Part model, mm, in its own coordinate system. A direction names the side the tool comes from. Round coordinates to 2 decimals unless told otherwise and drop trailing zeros. Loops run counter-clockwise (first coordinate to the right, second up) from the corner with the lowest first, then second, coordinate; pieces in that order, holes last. Notation, with made-up numbers: M -38,82 L 16,82 A29 cw 16,103 Z; hole C 41.5,27.5 d11. An arc over 180 degrees is marked long. Put each result on its own line as item: value. Start each with the question number.
1) Which spindle directions (+Z, -Z, +X, -X, +Y, -Y) get a long thin tool onto all of the face, cutting with end or side? Do faces 1 (the cylindrical face through (15.893, 0.211, 14.444)), 2 (the cylindrical face through (0, 26, 6)), 3 (the cylindrical face through (-15.893, 0.211, -14.444)). Say none if no direction does.
2) Pull direction Y, two halves, no side cores. Call faces 4 (the cylindrical face through (3, 0, -26)), 5 (the flat face through (0, 0, -33.5)), 6 (the cylindrical face through (15.918, 0.351, -14.444)): +Y half, -Y half, draft (parallel to the pull), parting line (faces both ways), or undercut.
3) Probe line 1 along Z through (x, y) = (9, 6.5); line 2 along Y through (x, z) = (-16.5, 18); line 3 along Y through (x, z) = (17.5, 14). List the from-to ranges inside material, lowest first.
4) Slice it at C-C on y = 23. Give the cut face in (x, z), then the cut area to 3 significant figures.
5) Slice it at B-B on z = -16. Give the cut face in (x, y), then the cut area to 3 significant figures.
6) Drop flat-ended pins along their axis: pin 1 Ø12 at (x, y) = (4.5, 20) entering from -Z; pin 2 Ø1 at (x, y) = (7.5, 14.5) entering from +Z; pin 3 Ø10 at (x, z) = (10.5, -3) entering from +Y; pin 4 Ø10 at (y, z) = (20.5, -27) entering from +X. Give the stop position or say it passes through.
7) Slice it at A-A on x = 0. Give the cut face in (y, z).
8) Slice it at D-D on z = -22. Give the cut face in (x, y).
Autodesk Inventor part; units mm, degrees
ref_plane "Arbeitsebene1" through (0, 25, 0) normal (0, 1, 0) x (-1, 0, 0)
ref_plane "YZ Plane" through (0, 0, 0) normal (1, 0, 0) x (0, 1, 0)
ref_plane "XY Plane" through (0, 0, 0) normal (0, 0, 1) x (1, 0, 0)
sketch "Skizze1" plane through (0, 0, 0) normal (0, 0, 1) x (1, 0, 0)
  circle A0 centre (0, 0) radius 25
  dimension "d0" = 50
extrude "Extrusion1" add sketch "Skizze1" along normal mid plane 37
sketch "Skizze2" plane through (0, 0, 18.5) normal (0, 0, 1) x (1, 0, 0)
  circle A0 centre (0, 0) radius 25
  circle A1 centre (0, 0) radius 3
  dimension "d3" = 6
extrude "Extrusion2" add sketch "Skizze2" along normal blind 6 contours A1
sketch "Skizze3" plane through (0, 0, -18.5) normal (0, 0, -1) x (-1, 0, 0)
  circle A0 centre (0, 0) radius 25
  circle A1 centre (0, 0) radius 3
  dimension "d6" = 6
extrude "Extrusion3" add sketch "Skizze3" along normal blind 15 contours A1
chamfer "Fase1" distance 0.5 angle 45 2 edges at (3, 0, -33.5) (-3, 0, 24.5)
sketch "Skizze4" plane through (0, 0, 18.5) normal (0, 0, 1) x (1, 0, 0)
  circle A0 centre (0, 0) radius 3
  line L0 (-17.5, 0) -> (17.5, 0) construction
  dimension "d12" = 35
hole "Bohrung1" at (-17.5, 0, 18.5) at (17.5, 0, 18.5) direction (0, 0, -1) diameter 3.242 depth 8 tip angle 118
mirror "Spiegeln1" about plane through (0, 0, 0) normal (0, 0, 1) of "Bohrung1"
ref_plane "Arbeitsebene1" through (0, 25, 0) normal (0, 1, 0) x (-1, 0, 0)
sketch "Skizze5" plane through (0, 25, 0) normal (0, 1, 0) x (-1, 0, 0)
  line L0 (-25, -18.5) -> (25, -18.5)
  line L1 (25, 18.5) -> (-25, 18.5)
  circle A0 centre (0, 3.5) radius 2.5
  point P0 (0, 0)
  dimension "d20" = 15
  dimension "d21" = 5
extrude "Extrusion4" add sketch "Skizze5" against normal blind 2 and the other way blind 2
properties part number "Tunel_Motor"
Recorded:
1. face 1: +Z
1. face 2: +Y
1. face 3: -Z
2. face 4: parting line
2. face 5: draft
2. face 6: undercut
3. line 1: z = -18.5 to 18.5
3. line 2: y = -18.78 to -1.28, 1.28 to 18.78
3. line 3: y = -17.85 to -1.62, 1.62 to 17.85
4. outline: M -9.8,-18.5 L 9.8,-18.5 L 9.8,18.5 L -9.8,18.5 Z
4. area: 725 mm2
5. outline: C 0,0 d50; hole C -17.5,0 d3.24; hole C 17.5,0 d3.24
5. area: 1,950 mm2
6. pin 1: stops at z = -18.5
6. pin 2: stops at z = 18.5
6. pin 3: stops at y = 24.39
6. pin 4: passes through
7. outline: M -25,-18.5 L -3,-18.5 L -3,-33 L -2.5,-33.5 L 2.5,-33.5 L 3,-33 L 3,-18.5 L 25,-18.5 L 25,1 L 27,1 L 27,6 L 25,6 L 25,18.5 L 3,18.5 L 3,24 L 2.5,24.5 L -2.5,24.5 L -3,24 L -3,18.5 L -25,18.5 Z
8. outline: C 0,0 d6
